Geometry: see drawing. Coordinates: mm, zero at the bounding-box minimum. A direction names the side the tool comes from. Coordinates: 2 decimals unless noted, no trailing zeros. Order: outer loops, then holes, each group sorted by start corner. A loop starts at its lowest first (then second) coordinate and runs counter-clockwise, first axis right, second up. Notation, with made-up numbers: M 20,5.5 L 31,5.5 A19 ccw 31,31.5 Z; hole C -32,-5 d11. An arc over 180 degrees is marked long. One line per item, written item: value.
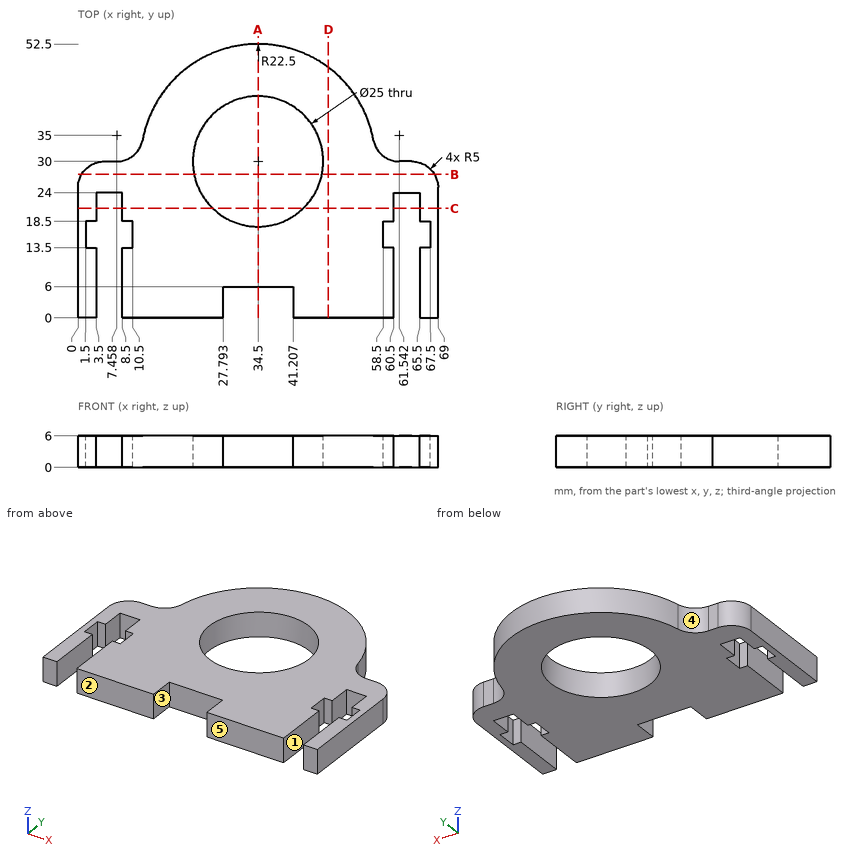
(1) Access query for the marked faces 1 and 2. Directions: +Z, -Z, +X, -X, +Y, -Y. A direction counts if a zero-diameter tool reaches every point of the face in a straight line with its end or side. Return the directions, or none.
Data:
face 1: +Z, -Z, -Y
face 2: +Z, -Z, +X, -X, -Y
(2) Ray query, line 1 (X direction, y = 9.5, z = 3.8); line 2 (X direction, y = 15, z = 1.15); line 3 (X direction, y = 4.5, z = 0.8). Return the intervals inside material, ascending. Write a range as from..to.
Data:
line 1: x = 0..3.5, 8.5..60.5, 65.5..69
line 2: x = 0..1.5, 10.5..58.5, 67.5..69
line 3: x = 0..3.5, 8.5..27.79, 41.21..60.5, 65.5..69
(3) Cut plane C-C on y = 21. Output: boundary loops of the cut face in (x, z) (1 decimal), plus the area to 3 significant figures.
Data:
outline: M 0,0 L 3.5,0 L 3.5,6 L 0,6 Z; M 8.5,0 L 25.8,0 L 25.8,6 L 8.5,6 Z; M 43.2,0 L 60.5,0 L 60.5,6 L 43.2,6 Z; M 65.5,0 L 69,0 L 69,6 L 65.5,6 Z
area: 250 mm2
(4) First-contact query: pin 1 (2 mm diameter, centred on y = 27.5, z = 1, fed in from +X); pin 2 (1.8 mm diameter, centred on x = 32.5, z = 1.5, fed in from -Y); pin 3 (3 mm diameter, centred on y = 22, z = 2.5, fed in from -X); pin 4 (2 mm diameter, centred on x = 66, z = 3.5, fed in from +Y). Flat tips, straight axial feed; report the tip coordinate or a pass-through.
Data:
pin 1: stops at x = 68.77
pin 2: stops at y = 6
pin 3: stops at x = 0
pin 4: stops at y = 29.9
(5) Cut plane A-A on x = 34.5. Output: boundary loops of the cut face in (y, z), plus the area to 3 significant figures.
Data:
outline: M 6,0 L 17.5,0 L 17.5,6 L 6,6 Z; M 42.5,0 L 52.5,0 L 52.5,6 L 42.5,6 Z
area: 129 mm2
(6) Cut plane B-B on y = 27.5. Output: boundary loops of the cut face in (x, z), plus the area to 3 significant figures.
Data:
outline: M 0.67,0 L 22.25,0 L 22.25,6 L 0.67,6 Z; M 46.75,0 L 68.33,0 L 68.33,6 L 46.75,6 Z
area: 259 mm2
(7) Draft query along X for the marked faces 3, 4 and 5. Return one class per face: released by +X, released by -X, zero draft, split by the parting line, or undercut.
Data:
face 3: undercut
face 4: released by -X
face 5: zero draft
(8) Cut plane D-D on x = 48. Output: boundary loops of the cut face in (y, z).
Data:
outline: M 0,0 L 48,0 L 48,6 L 0,6 Z
